The model under review builds one solid part; all positions refer to its coordinate system, in mm. A direction names the side the tool comes from. Coordinates: 2 decimals unless noted, no trailing zeros. Order: outer loops, then holes, each group sorted by start corner. A loop starts at its lowest first (then second) coordinate and runs counter-clockwise, first axis right, second up. Notation, with made-up numbers: (50, 32) -> (83, 32) arc R23 cw to (83, 48) -> close; hole circle Ø10 at (68.25, 18.25). An arc over 180 degrees is marked (long way). Put each result on its own line as item: value.
from build123d import *

# Parameters (mm, degrees)
ESBO_O1_W                  = 120
ESBO_O1_H                  = 120
RESSALTO_EXTRUS_O1_DEPTH   = 5
ESBO_O2_R                  = 16.75
CORTE_EXTRUS_O1_DEPTH      = 13
CORTE_EXTRUS_O2_DEPTH      = 28
CORTE_EXTRUS_O2_DEPTH_BACK = 29
ESBO_O3_R                  = 1.5
ESBO_O3_W                  = 22.9
ESBO_O3_H                  = 12.5
CORTE_EXTRUS_O3_DEPTH      = 32
CORTE_EXTRUS_O3_DEPTH_BACK = 28
ESBO_O4_R                  = 7.9


with BuildPart() as part:
    # Esboço1 → Ressalto-extrusão1 (new body)
    with BuildSketch(Plane.XY):
        with Locations((60, 60)):
            Rectangle(ESBO_O1_W, ESBO_O1_H)
    extrude(amount=RESSALTO_EXTRUS_O1_DEPTH)

    # Esboço2 → Corte-extrusão1 (cut)
    with BuildSketch(Plane.XY.offset(5)):
        with Locations((60, 60)):
            Circle(ESBO_O2_R)
    extrude(amount=-CORTE_EXTRUS_O1_DEPTH, mode=Mode.SUBTRACT)

    # Esboço3 → Corte-extrusão2 (cut, two sides: drawn at the far end of the back side and taken through both)
    with BuildSketch(Plane.XY.offset(-CORTE_EXTRUS_O2_DEPTH_BACK)):
        with Locations(Location((46.5, 19.48375, 0), (0, 0, 180))):
            Circle(ESBO_O3_R)
        with Locations(Location((73.566567065, 19.099645167, 0), (0, 0, 180))):
            Circle(ESBO_O3_R)
        with Locations((60.05, 19.48375)):
            Rectangle(ESBO_O3_W, ESBO_O3_H)
    extrude(amount=CORTE_EXTRUS_O2_DEPTH + CORTE_EXTRUS_O2_DEPTH_BACK, mode=Mode.SUBTRACT)

    # Esboço4 → Corte-extrusão3 (cut, two sides: drawn at the far end of the back side and taken through both)
    with BuildSketch(Plane.XY.offset(-CORTE_EXTRUS_O3_DEPTH_BACK)):
        with Locations(Location((47, 96.975019671, 0), (0, 0, 180))):
            Circle(ESBO_O4_R)
        with Locations(Location((73, 96.975019671, 0), (0, 0, 180))):
            Circle(ESBO_O4_R)
    extrude(amount=CORTE_EXTRUS_O3_DEPTH + CORTE_EXTRUS_O3_DEPTH_BACK, mode=Mode.SUBTRACT)


solid = part.part
Item 1: Consider section A-A on x = 60. Write out the cut boundary in (y, z), and give its area (3 significant figures).
Answers below:
outline: (0, 0) -> (13.23, 0) -> (13.23, 5) -> (0, 5) -> close; (25.73, 0) -> (43.25, 0) -> (43.25, 5) -> (25.73, 5) -> close; (76.75, 0) -> (120, 0) -> (120, 5) -> (76.75, 5) -> close
area: 370 mm^2
Item 2: For line 1 (Y direction, x = 60, z = 1); line 2 (Y direction, x = 47, z = 2.25); line 3 (X direction, y = 103, z = 3.35), list the stretches that pass through material, from the lowest coordinate up. Write a range as from..to.
Answers below:
line 1: 0..13.23, 25.73..43.25, 76.75..120
line 2: 0..18.07, 20.9..49.44, 70.56..89.08, 104.88..120
line 3: 0..41.89, 52.11..67.89, 78.11..120
Item 3: Consider section D-D on y = 24. Write out the cut boundary in (x, z).
Answers below:
outline: (0, 0) -> (48.6, 0) -> (48.6, 5) -> (0, 5) -> close; (71.5, 0) -> (120, 0) -> (120, 5) -> (71.5, 5) -> close
Item 4: Mouldability with a two-part tool opening along X and no side actions: class faces 3 (the cylindrical face through (65.465, 94.602, 2.465)), 4 (the flat face through (120, 59, 2)), 5 (the flat face through (59, 120, 2)) as +X half, -X half, draft (parallel to the pull), parting line (faces both ways), or undercut.
Answers below:
face 3: undercut
face 4: +X half
face 5: draft
Item 5: Consider section C-C on z = 1.6. Write out the cut boundary in (x, y).
Answers below:
outline: (0, 0) -> (120, 0) -> (120, 120) -> (0, 120) -> close; hole circle Ø15.8 at (47, 96.98); hole circle Ø33.5 at (60, 60); hole circle Ø3 at (46.5, 19.48); hole (48.6, 13.23) -> (71.5, 13.23) -> (71.5, 25.73) -> (48.6, 25.73) -> close; hole circle Ø15.8 at (73, 96.98); hole circle Ø3 at (73.57, 19.1)
Item 6: For faces 1 (the flat face through (59, 0, 2)), 2 (the flat face through (71.5, 19, 2)), list the 3-axis set-ups (+Z, -Z, +X, -X, +Y, -Y) from which the entire face can be reached by the end or side of a thin tool; tool diameter is ignored.
Answers below:
face 1: +Z, -Z, +X, -X, -Y
face 2: +Z, -Z
Item 7: Consider section B-B on y = 60. Write out the cut boundary in (x, z).
Answers below:
outline: (0, 0) -> (43.25, 0) -> (43.25, 5) -> (0, 5) -> close; (76.75, 0) -> (120, 0) -> (120, 5) -> (76.75, 5) -> close
